Geometry check sheet. Reference: the model listing, model coordinates, mm. Give positions to 0.01 mm unless a question says otherwise; leave off trailing zeros. Loops run counter-clockwise (first coordinate to the right, second up) from the corner with the lowest first, then second, coordinate; pieces in that order, holes last. Notation, with made-up numbers: (22, -10.5) -> (69, -10.5) arc R16 cw to (69, 6.5) -> close; hole circle Ø7 at (1, 66). An arc over 180 degrees is marked (long way). Write item = value, one per line.
```python
from build123d import *

# Parameters (mm, degrees)
SKETCH3_W          = 2.5
SKETCH3_H          = 82
SKETCH4_R          = 1
CUT_EXTRUDE1_DEPTH = 82
FILLET1_R          = 0.2


with BuildPart() as part:
    # Sketch3 → Revolve2 (revolve)
    with BuildSketch(Plane(origin=(0, 0, 0), x_dir=(0, 0, -1), z_dir=(1, 0, 0))):
        with Locations((1.25, 0)):
            Rectangle(SKETCH3_W, SKETCH3_H)
    revolve(axis=Axis((0, 41, 0), (0, -1, 0)))

    # Sketch4 → Cut-Extrude1 (cut)
    with BuildSketch(Plane(origin=(0, 41, 0), x_dir=(1, 0, 0), z_dir=(0, 1, 0))):
        Circle(SKETCH4_R)
    extrude(amount=-CUT_EXTRUDE1_DEPTH, mode=Mode.SUBTRACT)

    # Fillet1
    fillet1_edges = [part.edges().sort_by_distance(p)[0] for p in [
        (0, 41, 2.5),
        (0, -41, 2.5),
    ]]
    fillet(fillet1_edges, radius=FILLET1_R)


solid = part.part
```
Item 1: Section check B-B, the plane x = 0. Record the cut outline in (y, z).
Answer:
outline = (-41, -2.3) arc R0.2 ccw to (-40.8, -2.5) -> (40.8, -2.5) arc R0.2 ccw to (41, -2.3) -> (41, -1) -> (-41, -1) -> close; (-41, 1) -> (41, 1) -> (41, 2.3) arc R0.2 ccw to (40.8, 2.5) -> (-40.8, 2.5) arc R0.2 ccw to (-41, 2.3) -> close
Item 2: Section check C-C, the plane y = 14. Record the cut outline in (x, z), plus the area to 3 significant figures.
Answer:
outline = circle Ø5 at (0, 0); hole circle Ø2 at (0, 0)
area = 16.5 mm^2
Item 3: Draft check along Z on faces 1 (the cylindrical face through (0, 1, 1)), 2 (the cylindrical face through (-2.44, 0.57, 0.54)), 3 (the flat face through (1, -41, 1)). Enter one of: +Z half, -Z half, draft (parallel to the pull), parting line (faces both ways), or undercut.
Answer:
face_1 = undercut
face_2 = parting line
face_3 = draft
Item 4: Section check A-A, the plane z = 0. Record the cut outline in (x, y), plus the area to 3 significant figures.
Answer:
outline = (-2.5, -40.8) arc R0.2 ccw to (-2.3, -41) -> (-1, -41) -> (-1, 41) -> (-2.3, 41) arc R0.2 ccw to (-2.5, 40.8) -> close; (1, -41) -> (2.3, -41) arc R0.2 ccw to (2.5, -40.8) -> (2.5, 40.8) arc R0.2 ccw to (2.3, 41) -> (1, 41) -> close
area = 246 mm^2
Item 5: Thickness scan on L1, parallel to X at y = -11, z = 0; L2, parallel to Z at x = 0.2, y = -17; L3, parallel to Z at x = 0.7, y = -10.5. Record the ranges inside material, lowest first. Write a range as [from, to].
Answer:
L1 = [-2.5, -1], [1, 2.5]
L2 = [-2.49, -0.98], [0.98, 2.49]
L3 = [-2.4, -0.71], [0.71, 2.4]
Item 6: Gauge pin test, flat end, axial feed: pin 1 (2 mm diameter, centred on y = -16, z = -2, fed in from -X). Record the tip position at first contact, or that the pin passes through.
Answer:
pin_1 = -2.29
